Can you work these out from the model? Positions are in its coordinate system, mm. A direction names the side the tool comes from. Coordinates: 2 decimals unless noted, no trailing zeros. Write each loop counter-clockwise with the first axis right and the second up, starting at its lowest first coordinate (ties: lowest second). Pieces come first, ordered by that corner, then holes. Notation, with made-up numbers: (53.5, 77.5) -> (65.5, 77.5) arc R23 ccw to (65.5, 109.5) -> close; hole circle Ø11 at (1.25, 3). An arc over 180 degrees is marked (long way). Answer as CSV lines item,"result". Start each with the question number.
```python
from build123d import *

# Parameters (mm, degrees)
EJE_PROFILE_R         = 5
TUERCA_DCHA_PROFILE_R = 8.5
TUERCA_IZQ_PROFILE_R  = 8.5


with BuildPart() as part:
    # Eje: sweep along a curve in space
    with BuildLine() as eje_path:
        Line((-425.1, 65, -65), (-425.1, 65, 65))
    # Eje profile (on start of the path) → Eje (sweep)
    with BuildSketch(Plane(origin=(-425.1, 65, -65), x_dir=(1, 0, 0), z_dir=(0, 0, 1))):
        Circle(EJE_PROFILE_R)
    sweep(path=eje_path.line)

    # Tuerca_dcha: sweep along a curve in space
    with BuildLine() as tuerca_dcha_path:
        Line((-425.1, 65, 60), (-425.1, 65, 65))
    # Tuerca_dcha profile (on start of the path) → Tuerca_dcha (sweep)
    with BuildSketch(Plane(origin=(-425.1, 65, 60), x_dir=(1, 0, 0), z_dir=(0, 0, 1))):
        Circle(TUERCA_DCHA_PROFILE_R)
    sweep(path=tuerca_dcha_path.line)

    # Tuerca_izq: sweep along a curve in space
    with BuildLine() as tuerca_izq_path:
        Line((-425.1, 65, -65), (-425.1, 65, -60))
    # Tuerca_izq profile (on start of the path) → Tuerca_izq (sweep)
    with BuildSketch(Plane(origin=(-425.1, 65, -65), x_dir=(1, 0, 0), z_dir=(0, 0, 1))):
        Circle(TUERCA_IZQ_PROFILE_R)
    sweep(path=tuerca_izq_path.line)


solid = part.part
```
Q1. I need wall thicknesses on L1, parallel to Z at x = -429, y = 70.25; L2, parallel to Y at x = -423.5, z = 32; L3, parallel to X at y = 62.25, z = -33. Which ranges of each line are inside material? Lowest first, please.
Q2. Imagine slicing it at B-B (x = -425.1). Write out the boundary of the cut face in (y, z).
Q3. Which directions (+Z, -Z, +X, -X, +Y, -Y) give clear straight access to the entire face, cutting with the end or side of a thin tool? Please do faces 1 (the face through (-416.99, 67.55, -62.46)), 2 (the face through (-421, 61, 60)).
Q4. If we mould it in two halves opening along Z, with no side actions, what happens to faces 3 (the face through (-420.33, 66.5, 0.84)), 4 (the face through (-425, 65, 65)), 5 (the face through (-425, 65, -65))? For each: released by +Z, released by -Z, zero draft, split by the parting line, or undercut.
Q5. Imagine slicing it at A-A (y = 65). Write out the boundary of the cut face in (x, z).
Q6. For pin 1 (4 mm diameter, centred on x = -425.5, z = 19.5, fed in from +Y); pin 2 (1.5 mm diameter, centred on y = 60, z = -49.5, fed in from -X); pin 3 (4 mm diameter, centred on x = -424.5, z = -36.5, fed in from -Y); pin 4 (1 mm diameter, centred on x = -431.5, z = -18, fed in from -Y), each with a flat end and sliding along its axis, tell me the tip position at first contact or that it passes through.
Q7. Imagine slicing it at C-C (z = 48). Write out the boundary of the cut face in (x, y).
Entries:
1,L1,"-65 to -60, 60 to 65"
1,L2,"60.26 to 69.74"
1,L3,"-429.28 to -420.92"
2,outline,"(56.5, -65) -> (73.5, -65) -> (73.5, -60) -> (70, -60) -> (70, 60) -> (73.5, 60) -> (73.5, 65) -> (56.5, 65) -> (56.5, 60) -> (60, 60) -> (60, -60) -> (56.5, -60) -> close"
3,face 1,"+Z, -Z"
3,face 2,"none"
4,face 3,"undercut"
4,face 4,"released by +Z"
4,face 5,"released by -Z"
5,outline,"(-433.6, -65) -> (-416.6, -65) -> (-416.6, -60) -> (-420.1, -60) -> (-420.1, 60) -> (-416.6, 60) -> (-416.6, 65) -> (-433.6, 65) -> (-433.6, 60) -> (-430.1, 60) -> (-430.1, -60) -> (-433.6, -60) -> close"
6,pin 1,"y = 70"
6,pin 2,"x = -427.73"
6,pin 3,"y = 60"
6,pin 4,"through"
7,outline,"circle Ø10 at (-425.1, 65)"
